Verification items for the finished model (mm, model axes). A direction names the side the tool comes from. Give positions to 0.01 mm unless a question says otherwise; leave off trailing zeros. Order: outer loops, then holes, each group sorted by start corner. A loop starts at its lowest first (then second) coordinate and runs counter-clockwise, first axis right, second up. Notation, with made-up numbers: (47.25, -5) -> (97.25, -5) arc R20 ccw to (97.25, 3) -> close; hole circle Ø10 at (72, 56.5). An arc over 180 degrees is marked (long way). Return JSON: item names as keys, results as strings. Group by question number.
(1) Cross-section at B-B on z = 1.75. Enter the section's corners in (x, y), then the cut area to 3 significant figures.
(2) Tool access check on faces 1 (the face through (17, 27, 8)), 2 (the face through (17.167, 37.373, 1.479)). Record the directions out of +Z, -Z, +X, -X, +Y, -Y that give a thin tool (end or side, any length) a straight path to the whole face; none if there is none.
(3) Depth check by flat-ended pin: pin 1 Ø3 at (x, y) = (18.14, 29.94) entering from +Z; pin 2 Ø6 at (x, z) = (12, 2.5) entering from -Y; pin 3 Ø2 at (y, z) = (31.5, 3) entering from -X; pin 4 Ø1.9 at (x, y) = (19, 30) entering from +Z. Enter the tip coordinate at first touch or a pass-through.
(4) Thickness scan on line 1 along Z through (x, y) = (22.5, 30.75); line 2 along Y through (x, z) = (12.75, 7.25); line 3 along Y through (x, z) = (19, 8.5). Record the ranges inside material, lowest first.
(5) Cross-section at A-A on y = 31. State how many separate pieces and enclosed holes the cut face has, then the cut area to 3 significant figures.
(6) Cross-section at C-C on z = 10.75. Enter the section's corners in (x, y) (3 decimals), then the cut area to 3 significant figures.
(7) Release check for a two-part mould opening along Y. For faces 3 (the face through (12.503, 30.185, 9.181)), 4 (the face through (13.506, 29.278, 6.182)), 5 (the face through (15, 31, 13)) record: pulls with the +Y half, pulls with the -Y half, needs draft (parallel to the pull), parting line crosses it, or undercut.
from build123d import *

# Parameters (mm, degrees)
SKETCH_6_R               = 7.5
EXTRUDE_1_DEPTH          = 3
SKETCH_7_R               = 4.5
SKETCH_7_R_2             = 3.15
EXTRUDE_2_DEPTH          = 10
SKETCH_9_R               = 1.65
CUT_EXTRUDE_1_DEPTH      = 3
CHAMFER_1_SIZE           = 3
CHAMFER_1_SIZE_2         = 10
CUT_EXTRUDE_2_DEPTH      = 37.903513147
CUT_EXTRUDE_2_DEPTH_BACK = 37.903513147
SKETCH_10_R              = 1.35


with BuildPart() as part:
    # 草图6 → 凸台-拉伸1 (new body)
    with BuildSketch(Plane.XY):
        with Locations((18.143108258, 29.936835998)):
            Circle(SKETCH_6_R)
    extrude(amount=EXTRUDE_1_DEPTH)

    # 草图7 → 凸台-拉伸2 (add)
    with BuildSketch(Plane.XY.offset(3)):
        with Locations((18.143108258, 29.936835998)):
            Circle(SKETCH_7_R)
        with Locations((18.143108258, 29.936835998)):
            Circle(SKETCH_7_R_2, mode=Mode.SUBTRACT)
    extrude(amount=EXTRUDE_2_DEPTH)

    # 草图9 → 切除-拉伸1 (cut)
    with BuildSketch(Plane.XY.offset(3)):
        with Locations((18.143108258, 29.936835998)):
            Circle(SKETCH_9_R)
    extrude(amount=-CUT_EXTRUDE_1_DEPTH, mode=Mode.SUBTRACT)

    # 倒角1
    # the kernel refuses this chamfer: 10, 3 mm, written as the material it adds along each edge
    with BuildSketch(Plane(origin=(18.143108258, 29.936835998, 3), x_dir=(1, 0, 0), z_dir=(0, -1, 0))) as chamfer_1_piece_1_section:
        Polygon((4.5 + CHAMFER_1_SIZE, 0), (4.5, CHAMFER_1_SIZE_2), (4.5, 0), align=None)
    chamfer_1_piece_1 = revolve(axis=Axis((18.143108258, 29.936835998, 3), (0, 0, 1)), mode=Mode.PRIVATE)
    chamfer_1_piece_1 = chamfer_1_piece_1 & Plane(origin=(18.143108258, 29.936835998, 7.975650117), x_dir=(1, 0, 0), z_dir=(0, 0, -1)) * Cylinder(7.5, 40, mode=Mode.PRIVATE)
    chamfer_1_piece_1 = split(chamfer_1_piece_1, bisect_by=Plane(origin=(12.224274533, 29.936835998, 13), z_dir=(0, 0, -1)), keep=Keep.TOP, mode=Mode.PRIVATE)
    add(chamfer_1_piece_1)

    # 草图10 → 切除-拉伸2 (cut, two sides: drawn at the far end of the back side and taken through both)
    with BuildSketch(Plane(origin=(18.921476442, 3.905687751, 0), x_dir=(0, 0, 1), z_dir=(-0.9793537694565077, -0.20215388754938593, 0)).offset(-CUT_EXTRUDE_2_DEPTH_BACK)):
        with Locations(Location((7.5, 25.651053313, 0), (0, 0, 270))):
            Circle(SKETCH_10_R)
    extrude(amount=CUT_EXTRUDE_2_DEPTH + CUT_EXTRUDE_2_DEPTH_BACK, mode=Mode.SUBTRACT)


solid = part.part
Verdict:
{
 "1": {"outline": "circle Ø15 at (18.14, 29.94); hole circle Ø3.3 at (18.14, 29.94)", "area": "168 mm²"},
 "2": {"face 1": "+Z", "face 2": "+Z, -Z"},
 "3": {"pin 1": "through", "pin 2": "y = 23.13", "pin 3": "x = 10.66", "pin 4": "z = 3"},
 "4": {"line 1": "0 to 6.15, 8.85 to 13", "line 2": "26.83 to 27.47, 30.18 to 33.05", "line 3": "24.15 to 26.91, 32.97 to 35.72"},
 "5": {"separate pieces": "3", "enclosed holes": "0", "area": "87.5 mm²"},
 "6": {"outline": "circle Ø10.35 at (18.143, 29.937); hole circle Ø6.3 at (18.143, 29.937)", "area": "53.0 mm²"},
 "7": {"face 3": "parting line crosses it", "face 4": "undercut", "face 5": "needs draft"}
}
